from build123d import *

# Parameters (mm, degrees)
BOSS_EXTRUDE1_DEPTH     = 16
SKETCH2_W               = 22
SKETCH2_H               = 15
CUT_EXTRUDE1_DEPTH      = 12
CUT_EXTRUDE2_DEPTH      = 94.037626797
CUT_EXTRUDE2_DEPTH_BACK = 12
CUT_EXTRUDE4_DEPTH      = 12
CUT_EXTRUDE5_DEPTH      = 94.037626797


with BuildPart() as part:
    # Sketch1 → Boss-Extrude1 (new body)
    with BuildSketch(Plane(origin=(0, 0, 0), x_dir=(1, 0, 0), z_dir=(0, 1, 0))):
        Polygon((69.282032303, 0), (34.641016151, 60), (-34.641016151, 60), (-69.282032303, 0), (-34.641016151, -60), (34.641016151, -60), align=None)
    extrude(amount=BOSS_EXTRUDE1_DEPTH)

    # Sketch2 → Cut-Extrude1 (cut)
    with BuildSketch(Plane(origin=(0, 16, 0), x_dir=(1, 0, 0), z_dir=(0, 1, 0))):
        with Locations((-18.641016151, 52.5)):
            Rectangle(SKETCH2_W, SKETCH2_H)
        with Locations((18.641016151, 52.5)):
            Rectangle(SKETCH2_W, SKETCH2_H)
        Polygon((66.782032303, -4.330127019), (53.791651246, 3.169872981), (42.791651246, -15.882685902), (55.782032303, -23.382685902), align=None)
        Polygon((48.141016151, -36.617314098), (35.150635095, -29.117314098), (24.150635095, -48.169872981), (37.141016151, -55.669872981), align=None)
        Polygon((-37.141016151, -55.669872981), (-24.150635095, -48.169872981), (-35.150635095, -29.117314098), (-48.141016151, -36.617314098), align=None)
        Polygon((-55.782032303, -23.382685902), (-42.791651246, -15.882685902), (-53.791651246, 3.169872981), (-66.782032303, -4.330127019), align=None)
    extrude(amount=-CUT_EXTRUDE1_DEPTH, mode=Mode.SUBTRACT)

    # Sketch3 → Cut-Extrude2 (cut, two sides: drawn at the far end of the back side and taken through both)
    with BuildSketch(Plane(origin=(0, 16, 0), x_dir=(1, 0, 0), z_dir=(0, 1, 0)).offset(-CUT_EXTRUDE2_DEPTH_BACK)):
        Polygon((-43.560889132, -5.4496732), (17.060889132, -40.4496732), (43.560889132, 5.4496732), (-17.060889132, 40.4496732), align=None)
        Polygon((-22.060889132, 31.789419162), (-28.060889132, 21.397114317), (-49.711524227, 33.897114317), (-43.711524227, 44.289419162), align=None)
    extrude(amount=CUT_EXTRUDE2_DEPTH + CUT_EXTRUDE2_DEPTH_BACK, mode=Mode.SUBTRACT)

    # Sketch4 → Cut-Extrude4 (cut)
    with BuildSketch(Plane(origin=(0, 16, 0), x_dir=(1, 0, 0), z_dir=(0, 1, 0))):
        Polygon((-53.791651246, 3.169872981), (-59.853829072, -0.330127019), (-64.663230149, 8), (-60.621778265, 15), align=None)
        Polygon((-24.150635095, -48.169872981), (-30.212812921, -51.669872981), (-25.403411844, -60), (-17.320508076, -60), align=None)
        Polygon((43.301270189, 45), (29.641016151, 45), (29.641016151, 52), (39.259818305, 52), align=None)
        Polygon((-43.301270189, 45), (-29.641016151, 45), (-29.641016151, 52), (-39.259818305, 52), align=None)
        Polygon((17.320508076, -60), (24.150635095, -48.169872981), (30.212812921, -51.669872981), (25.403411844, -60), align=None)
        Polygon((60.621778265, 15), (53.791651246, 3.169872981), (59.853829072, -0.330127019), (64.663230149, 8), align=None)
    extrude(amount=-CUT_EXTRUDE4_DEPTH, mode=Mode.SUBTRACT)

    # Sketch7 → Cut-Extrude5 (cut, through all)
    with BuildSketch(Plane(origin=(0, 16, 0), x_dir=(1, 0, 0), z_dir=(0, 1, 0))):
        Polygon((-41.880108514, -10.461524227), (-15.299782134, -56.5), (15.299782134, -56.5), (20.940054257, -46.730762114), align=None)
        Polygon((-11.880108514, 41.5), (50.940054257, 5.230762114), (56.580326381, 15), (41.280544247, 41.5), align=None)
    extrude(amount=-CUT_EXTRUDE5_DEPTH, mode=Mode.SUBTRACT)


solid = part.part
Here's how the part is built. I have some questions about the finished solid (model axes, mm). A direction names the side the tool comes from. Coordinates: 2 decimals unless noted, no trailing zeros. Write each loop counter-clockwise with the first axis right and the second up, starting at its lowest first coordinate (ties: lowest second). Pieces come first, ordered by that corner, then holes.
Item 1: Will these pins go through, and if not, where does the flat tip stop? pin 1 (1 mm diameter, centred on y = 2, z = -6.5, fed in from -X); pin 2 (19 mm diameter, centred on x = -53.5, z = 1, fed in from +Y); pin 3 (2 mm diameter, centred on x = -54, z = 17.5, fed in from +Y); pin 4 (5 mm diameter, centred on y = 7, z = -7, fed in from +X).
Item 2: I want a section at B-B on x = 2.5. Write out the boundary of the cut face in (y, z), and give its area (3 significant figures).
Item 3: If I drill on line 1 (X direction, y = 12.25, z = 39); line 2 (X direction, y = 14.75, z = 26.5); line 3 (Z direction, x = -3.5, y = 15.75), over which ranges is the centre line in solid material (lowest first)?
Item 4: On a 3-axis mill with a long thin cutter (end or side, diameter ignored), from which of +Z, -Z, +X, -X, +Y, -Y can I reach the whole of each face in a straight line? I mean faces 4 (the flat face through (49.196, 10.084, 19.58)), 5 (the flat face through (-33.73, 10.08, 53.7)), 6 (the flat face through (62.225, 10.084, -3.777)), 7 (the flat face through (0, 6, -60)), 8 (the flat face through (-28.776, 8.112, 33.158)). Say none if no direction works.
Item 5: If we mould it in two halves opening along Z, with no side actions, what happens to faces 1 (the flat face through (51.72, 6.11, 30.42)), 2 (the flat face through (-65, 16, -1)), 3 (the flat face through (-4, 4, -3))? For each: +Z half, -Z half, draft (parallel to the pull), parting line (faces both ways), or undercut.
Item 6: I want a section at A-A on y = 2.5. Write out the boundary of the cut face in (x, z).
Item 7: I want a section at C-C on y = 13.5. Count the separate pieces of the cut face and the enclosed holes in it, and give its area (3 significant figures).
Findings below:
1. pin 1: stops at x = -65.82
1. pin 2: stops at y = 16
1. pin 3: stops at y = 4
1. pin 4: stops at x = 66.68
2. outline: (0, -60) - (16, -60) - (16, -41.5) - (0, -41.5) - close; (0, -33.2) - (16, -33.2) - (16, -29.16) - (4, -29.16) - (4, 32.04) - (16, 32.04) - (16, 36.08) - (0, 36.08) - close; (0, 56.5) - (16, 56.5) - (16, 60) - (0, 60) - close
2. area: 726 mm2
3. line 1: x = -29.44 to -25.4, 7.55 to 14.55, 17.9 to 29.44
3. line 2: x = -53.98 to -32.62, -14.1 to -7.1, 25.11 to 53.98
3. line 3: z = -60 to -41.5, -36.66 to -32.62, 28.58 to 32.62, 56.5 to 60
4. face 4: +X, +Y
4. face 5: -X, +Y
4. face 6: +Y
4. face 7: -Z, +X, -X, +Y, -Y
4. face 8: +Y, -Y
5. face 1: +Z half
5. face 2: draft
5. face 3: undercut
6. outline: (-69.28, 0) - (-34.64, -60) - (34.64, -60) - (69.28, 0) - (34.64, 60) - (-34.64, 60) - close; hole (-41.88, 10.46) - (20.94, 46.73) - (15.3, 56.5) - (-15.3, 56.5) - close; hole (-11.88, -41.5) - (41.28, -41.5) - (56.58, -15) - (50.94, -5.23) - close
7. separate pieces: 7
7. enclosed holes: 2
7. area: 3,760 mm2
